Design review of the part built by this model. Coordinates are the model's own, in mm. Face numbers are marked on the shaded views. A direction names the side the tool comes from. Coordinates: 2 decimals unless noted, no trailing zeros. Loops run counter-clockwise (first coordinate to the right, second up) from the corner with the lowest first, then second, coordinate; pieces in that order, holes last. Notation, with made-up numbers: M 89,44.5 L 112,44.5 A24 ccw 112,68.5 Z; hole C 73.25,31.5 d8. An arc over 180 degrees is marked long. Put each result on its own line as item: value. Start each with the question number.
(1) Take a section at C-C, the plane z = -0.5. Give the boundary of the cut face in (x, y), then the cut area to 3 significant figures.
(2) Clearance check with flat-ended pins moving along their axes: pin 1 (6.5 mm diameter, centred on x = 69, y = 7, fed in from -Z) (3 decimals); pin 2 (2 mm diameter, centred on y = 3.5, z = -18, fed in from +X); pin 3 (10.5 mm diameter, centred on x = -49, z = -16.5, fed in from +Y); pin 4 (12 mm diameter, centred on x = 49.21, y = 4.19, fed in from -Z) (3 decimals). State where each tip first meets the part, or that it passes through.
(3) Take a section at B-B, the plane x = -49.5. Give the boundary of the cut face in (y, z).
(4) The part is to be moulded in two halves that separate along X. For the marked faces 1, 2 and 3, say which applies: +X half, -X half, draft (parallel to the pull), parting line (faces both ways), or undercut.
(5) Take a section at A-A, the plane y = -11. Give the boundary of the cut face in (x, z) (3 decimals), then the cut area to 3 significant figures.
(6) For the marked faces 4, 5, 6, 7 and 8, list the 3-axis set-ups (+Z, -Z, +X, -X, +Y, -Y) from which the entire face can be reached by the end or side of a thin tool; tool diameter is ignored.
(7) Take a section at D-D, the plane z = 13. Give the boundary of the cut face in (x, y).
(8) For probe 1 along X at (y, z) = (0, 21.5); probe 2 along Y at (x, z) = (-57, -4.5); probe 3 along Z at (x, y) = (67, 17) (3 decimals), list the stretches that pass through material, from the lowest coordinate up. Write a range as [from, to].
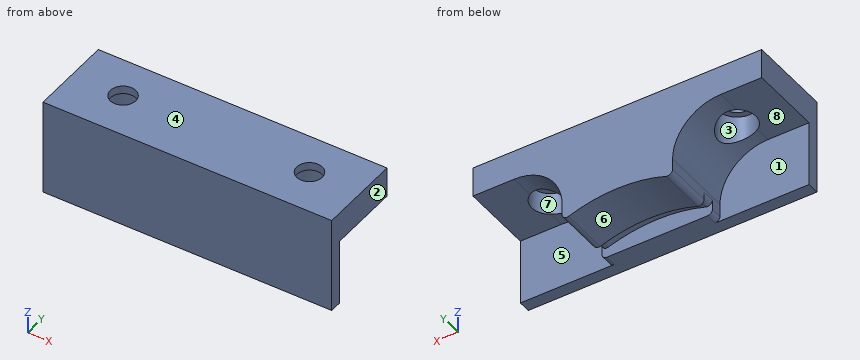
```python
from build123d import *

# Parameters (mm, degrees)
BOSS_EXTRUDE1_DEPTH     = 25.4
BOSS_EXTRUDE2_DEPTH     = 6.604
SKETCH3_W               = 152.4
SKETCH3_H               = 50.8
BOSS_EXTRUDE3_DEPTH     = 12.446
SKETCH5_W               = 47.049242613
SKETCH5_H               = 34.925
CUT_EXTRUDE1_DEPTH      = 38.1
FILLET1_R               = 2.54
FILLET2_R               = 25.4
CUT_EXTRUDE2_DEPTH      = 11.6332
CUT_EXTRUDE2_DEPTH_BACK = 85.242269675
CUT_EXTRUDE2_START      = 9.525
SKETCH6_R               = 9.9187
SKETCH7_R               = 6.7437
CUT_EXTRUDE3_DEPTH      = 93.840002113


with BuildPart() as part:
    # Sketch1 → Boss-Extrude1 (new body)
    with BuildSketch(Plane(origin=(0, 0, 0), x_dir=(1, 0, 0), z_dir=(0, 1, 0))):
        with BuildLine():
            Line((76.2, -25.4), (76.2, 25.4))
            Line((76.2, 25.4), (29.150757387, 25.4))
            ThreePointArc((29.150757387, 25.4), (0, 19.601553837), (-29.150757387, 25.4))
            Line((-29.150757387, 25.4), (-76.2, 25.4))
            Line((-76.2, 25.4), (-76.2, -25.4))
            Line((-76.2, -25.4), (76.2, -25.4))
        make_face()
    extrude(amount=BOSS_EXTRUDE1_DEPTH)

    # Sketch2 → Boss-Extrude2 (add)
    with BuildSketch(Plane.XZ):
        with BuildLine():
            Line((-76.2, 25.4), (76.2, 25.4))
            Line((76.2, 25.4), (76.2, -21.59))
            Line((76.2, -21.59), (29.966893046, -21.59))
            ThreePointArc((29.966893046, -21.59), (0, -15.766153837), (-29.966893046, -21.59))
            Line((-29.966893046, -21.59), (-76.2, -21.59))
            Line((-76.2, -21.59), (-76.2, 25.4))
        make_face()
    extrude(amount=BOSS_EXTRUDE2_DEPTH)

    # Sketch3 → Boss-Extrude3 (add)
    with BuildSketch(Plane.XZ.offset(6.604)):
        Rectangle(SKETCH3_W, SKETCH3_H)
    extrude(amount=BOSS_EXTRUDE3_DEPTH)

    # Sketch5 → Cut-Extrude1 (cut)
    with BuildSketch(Plane(origin=(0, 25.4, 0), x_dir=(1, 0, 0), z_dir=(0, 1, 0))):
        with Locations((-52.675378694, 7.9375)):
            Rectangle(SKETCH5_W, SKETCH5_H)
        with Locations((52.675378694, 7.9375)):
            Rectangle(SKETCH5_W, SKETCH5_H)
    extrude(amount=-CUT_EXTRUDE1_DEPTH, mode=Mode.SUBTRACT)

    # Fillet1
    fillet1_edges = [part.edges().sort_by_distance(p)[0] for p in [
        (29.150757387, 12.7, -25.4),
        (-29.150757387, 12.7, -25.4),
        (-29.150757387, -9.652, -25.4),
        (-29.150757387, -3.302, -21.265527456),
        (29.150757387, -9.652, -25.4),
        (29.150757387, -3.302, -21.265527456),
    ]]
    fillet(fillet1_edges, radius=FILLET1_R)

    # Fillet2
    fillet2_edges = [part.edges().sort_by_distance(p)[0] for p in [
        (-29.150757387, 6.35, 9.525),
        (29.150757387, 6.35, 9.525),
    ]]
    fillet(fillet2_edges, radius=FILLET2_R)

    # Sketch6 → Cut-Extrude2 (cut, two sides: drawn at the far end of the back side and taken through both)
    with BuildSketch(Plane.XY.offset(CUT_EXTRUDE2_START - CUT_EXTRUDE2_DEPTH_BACK)):
        with Locations(Location((49.2125, 4.191, 0), (0, 0, 302.561278337))):
            Circle(SKETCH6_R)
        with Locations(Location((-49.2125, 4.191, 0), (0, 0, 237.438721663))):
            Circle(SKETCH6_R)
    extrude(amount=CUT_EXTRUDE2_DEPTH + CUT_EXTRUDE2_DEPTH_BACK, mode=Mode.SUBTRACT)

    # Sketch7 → Cut-Extrude3 (cut, through all)
    with BuildSketch(Plane(origin=(0, 0, 21.1582), x_dir=(-1, 0, 0), z_dir=(0, 0, -1))):
        with Locations((-49.2125, 4.191)):
            Circle(SKETCH7_R)
        with Locations((49.2125, 4.191)):
            Circle(SKETCH7_R)
    extrude(amount=-CUT_EXTRUDE3_DEPTH, mode=Mode.SUBTRACT)


solid = part.part
```
Computed values:
1. outline: M -76.2,-19.05 L 76.2,-19.05 L 76.2,-12.7 L 34.33,-12.7 L 34.33,25.4 L -34.33,25.4 L -34.33,-12.7 L -76.2,-12.7 Z
1. area: 3,580 mm^2
2. pin 1: stops at z = 9.525
2. pin 2: stops at x = 29.15
2. pin 3: stops at y = -12.7
2. pin 4: passes through
3. outline: M -19.05,-25.4 L -12.7,-25.4 L -12.7,9.02 L -5.72,9.02 L -5.72,21.16 L -2.55,21.16 L -2.55,25.4 L -19.05,25.4 Z; M 10.93,21.16 L 14.11,21.16 L 14.11,9.02 L 25.4,9.02 L 25.4,25.4 L 10.93,25.4 Z
4. face 1: draft
4. face 2: +X half
4. face 3: undercut
5. outline: M -76.2,9.525 L -54.551,9.525 A25.4 cw -29.151,-15.875 L -29.151,-22.86 A2.54 ccw -26.611,-25.4 L 26.611,-25.4 A2.54 ccw 29.151,-22.86 L 29.151,-15.875 A25.4 cw 54.551,9.525 L 76.2,9.525 L 76.2,25.4 L -76.2,25.4 Z
5. area: 4,730 mm^2
6. face 4: +Z, +X, -X, +Y, -Y
6. face 5: -Z, +X, +Y
6. face 6: -Z, +Y
6. face 7: -Z
6. face 8: -Z, -X, +Y
7. outline: M -76.2,-19.05 L 76.2,-19.05 L 76.2,25.4 L -76.2,25.4 Z; hole C -49.21,4.19 d19.84; hole C 49.21,4.19 d19.84
8. probe 1: x = [-76.2, -54.5], [-43.93, 43.93], [54.5, 76.2]
8. probe 2: y = [-19.05, -12.7]
8. probe 3: z = [9.525, 25.4]
